```python
from build123d import *

# Parameters (mm, degrees)
F0_R     = 35.56
F0_R_2   = 30.7975
F1_DEPTH = 63.5
F2_R     = 43.18
F2_R_2   = 35.56
F2_R_3   = 30.7975
F3_DEPTH = 6.35
F4_R     = 35.56
F4_R_2   = 30.7975
F5_DEPTH = 38.1
F7_DEPTH = 63.5
F9_DEPTH = 6.35


with BuildPart() as f1:
    # F0 (on Front) → F1 (new body)
    with BuildSketch(Plane.XZ):
        Circle(F0_R)
        Circle(F0_R_2, mode=Mode.SUBTRACT)
    extrude(amount=F1_DEPTH)

    # F2 (on face) → F3 (join)
    with BuildSketch(Plane.XZ.offset(63.5)):
        Circle(F2_R)
        Circle(F2_R_2, mode=Mode.SUBTRACT)
        Circle(F2_R_2)
        Circle(F2_R_3, mode=Mode.SUBTRACT)
    extrude(amount=F3_DEPTH)

    # F4 (on face) → F5 (join)
    with BuildSketch(Plane.XZ.offset(69.85)):
        Circle(F4_R)
        Circle(F4_R_2, mode=Mode.SUBTRACT)
    extrude(amount=F5_DEPTH)

    # F6 (on face) → F7 (cut, through all)
    with BuildSketch(Plane(origin=(0, 0, 0), x_dir=(-1, 0, 0), z_dir=(0, 1, 0))):
        with BuildLine():
            Line((26.6714173731, -15.39875), (0, 0))
            Line((0, 0), (-26.6714173731, -15.39875))
            ThreePointArc((-26.6714173731, -15.39875), (0, -30.7975), (26.6714173731, -15.39875))
        make_face()
        with BuildLine():
            ThreePointArc((26.6714173731, -15.39875), (0, -30.7975), (-26.6714173731, -15.39875))
            Line((-26.6714173731, -15.39875), (-30.7958633586, -17.78))
            ThreePointArc((-30.7958633586, -17.78), (0, -35.56), (30.7958633586, -17.78))
            Line((30.7958633586, -17.78), (26.6714173731, -15.39875))
        make_face()
        with BuildLine():
            ThreePointArc((30.7958633586, -17.78), (0, -35.56), (-30.7958633586, -17.78))
            Line((-30.7958633586, -17.78), (-66.8170764648, -38.5768570834))
            Line((-66.8170764648, -38.5768570834), (66.8170764648, -38.5768570834))
            Line((66.8170764648, -38.5768570834), (30.7958633586, -17.78))
        make_face()
    extrude(amount=-F7_DEPTH, mode=Mode.SUBTRACT)

    # F8 (on face) → F9 (cut, through all)
    with BuildSketch(Plane(origin=(0, -63.5, 0), x_dir=(-1, 0, 0), z_dir=(0, 1, 0))):
        with BuildLine():
            Line((30.7958633586, -17.78), (26.6714173731, -15.39875))
            ThreePointArc((26.6714173731, -15.39875), (0, -30.7975), (-26.6714173731, -15.39875))
            Line((-26.6714173731, -15.39875), (-30.7958633586, -17.78))
            Line((-30.7958633586, -17.78), (-37.3949769354, -21.59))
            ThreePointArc((-37.3949769354, -21.59), (0, -43.18), (37.3949769354, -21.59))
            Line((37.3949769354, -21.59), (30.7958633586, -17.78))
        make_face()
    extrude(amount=-F9_DEPTH, mode=Mode.SUBTRACT)


solid = f1.part
```
Part model, mm, in its own coordinate system. A direction names the side the tool comes from. Coordinates: 2 decimals unless noted, no trailing zeros. Order: outer loops, then holes, each group sorted by start corner. A loop starts at its lowest first (then second) coordinate and runs counter-clockwise, first axis right, second up. Notation, with made-up numbers: (1.5, 24) -> (11.5, 24) arc R15 cw to (11.5, 42) -> close; hole circle Ø6 at (5, 71.5). An arc over 180 degrees is marked (long way). Put each result on its own line as item: value. Start each with the question number.
(1) Band-saw the part on B-B (x = 0). Give the cut face in (y, z).
(2) Probe line 1 along X through (y, z) = (-61, 0); line 2 along Z through (x, y) = (-28.5, -48); line 3 along X through (y, z) = (-89, 6.5). List the from-to ranges inside material, lowest first. Write a range as [from, to].
(3) Band-saw the part on C-C (y = -94.5). Give the cut face in (x, z) (1 decimal).
(4) Band-saw the part on D-D (x = -24). Give the cut face in (y, z).
(5) Mould opens along X. For faces 1 (the face through (-3, -69.85, 37)), 2 (the face through (-4.009, -53.219, 30.535)), 3 (the face through (1.043, -31.306, 35.545)) say: pulls with the +X half, pulls with the -X half, needs draft (parallel to the pull), parting line crosses it, or undercut.
(6) Which spindle directions (+Z, -Z, +X, -X, +Y, -Y) get a long thin tool onto all of the face, cutting with end or side? Do faces 4 (the face through (2, 0, 31)), 5 (the face through (-7.709, -88.633, -34.714)), 6 (the face through (0, -69.85, -31)). Say none if no direction does.
(7) Band-saw the part on A-A (z = 0). Give the cut face in (x, y).
(8) Pin check, flat tips, straight feed: pin 1 Ø10 at (x, y) = (14.5, -91.5) entering from +Z; pin 2 Ø12 at (x, y) = (20, -81.5) entering from -Z; pin 3 Ø2 at (y, z) = (-42.5, -16.5) entering from -X. Stop position of each tip, or through.
Determined:
1. outline: (-107.95, -35.56) -> (-69.85, -35.56) -> (-69.85, -30.8) -> (-107.95, -30.8) -> close; (-107.95, 30.8) -> (0, 30.8) -> (0, 35.56) -> (-63.5, 35.56) -> (-63.5, 43.18) -> (-69.85, 43.18) -> (-69.85, 35.56) -> (-107.95, 35.56) -> close
2. line 1: x = [-35.56, -30.8], [30.8, 35.56]
2. line 2: z = [-16.45, -11.67], [11.67, 21.27]
2. line 3: x = [-34.96, -30.1], [30.1, 34.96]
3. outline: circle Ø71.1 at (0, 0); hole circle Ø61.6 at (0, 0)
4. outline: (-107.95, -26.24) -> (-69.85, -26.24) -> (-69.85, -19.3) -> (-107.95, -19.3) -> close; (-107.95, 19.3) -> (0, 19.3) -> (0, 26.24) -> (-63.5, 26.24) -> (-63.5, 35.9) -> (-69.85, 35.9) -> (-69.85, 26.24) -> (-107.95, 26.24) -> close
5. face 1: needs draft
5. face 2: undercut
5. face 3: parting line crosses it
6. face 4: +Z, -Z, +X, -X, +Y
6. face 5: -Y
6. face 6: -Z, +Y
7. outline: (-43.18, -69.85) -> (-35.56, -69.85) -> (-35.56, -107.95) -> (-30.8, -107.95) -> (-30.8, 0) -> (-35.56, 0) -> (-35.56, -63.5) -> (-43.18, -63.5) -> close; (30.8, -107.95) -> (35.56, -107.95) -> (35.56, -69.85) -> (43.18, -69.85) -> (43.18, -63.5) -> (35.56, -63.5) -> (35.56, 0) -> (30.8, 0) -> close
8. pin 1: stops at z = 34.27
8. pin 2: stops at z = -32.69
8. pin 3: stops at x = -32
